Autodesk Fusion 360 part; units mm, degrees
sketch "Sketch1" plane through (0, 0, 0) normal (0, 0, 1) x (1, 0, 0)
  line L0 (7.5, 9) -> (-7.5, 9)
  line L1 (-7.5, 9) -> (-7.5, -9)
  line L2 (-7.5, -9) -> (2.5, -9)
  line L3 (7.5, -3) -> (7.5, 7)
  line L4 (2.5, -9) -> (7.5, -3)
  line L5 (5.5, 7) -> (7.5, 9)
  line L6 (7.5, 7) -> (7.5, 9)
  line L7 (5.5, 7) -> (-7.5, 7)
  dimension "d2" = 18
  dimension "d3" = 10
  dimension "d4" = 2
  dimension "d5" = 2
extrude "Extrude1" add sketch "Sketch1" along normal blind 6 contours L1 L2 L3 L4 L5 L6 L7
sketch "Sketch2" plane through (0, 0, 6) normal (0, 0, 1) x (-1, 0, 0)
  line L0 (-5.5, -7) -> (7.5, -7)
  line L1 (7.5, -7) -> (7.5, 9)
  line L2 (7.5, 9) -> (-2.5, 9)
  line L3 (-2.5, 9) -> (-7.5, 3)
  line L4 (-7.5, 3) -> (-7.5, -9)
  line L5 (-7.5, -9) -> (-5.5, -7)
  line L6 (-7.5, -9) -> (7.5, -9)
  line L7 (7.5, -9) -> (7.5, -7)
  dimension "d8" = 15
extrude "Extrude2" add sketch "Sketch2" along normal blind 6 and the other way blind 6 contours L0 L5 L6 L7
extrude "Extrude3" add 1 faces at (-2.5, 9, 6) along direction (0, 1, 0) blind 2
sketch "Sketch3" plane through (0, 7, 0) normal (0, -1, 0) x (1, 0, 0)
  line L0 (-7.5, 6) -> (5.5, 6)
  line L1 (5.5, 6) -> (5.5, 12)
  line L2 (5.5, 12) -> (-7.5, 12)
  line L3 (-7.5, 12) -> (-7.5, 6)
  line L4 (5.5, 12) -> (5.5, 10) construction
  line L5 (5.5, 10) -> (-0.5, 10) construction
  line L6 (-0.5, 10) -> (-7.5, 10)
  line L7 (-0.5, 10) -> (-0.5, 6)
extrude "Extrude4" add sketch "Sketch3" along normal blind 16 contours L0 L3 L6 L7
sketch "Sketch4" plane through (0, 0, 10) normal (0, 0, 1) x (-1, 0, 0)
  line L0 (0.5, -7) -> (7.5, -7)
  line L1 (7.5, -7) -> (7.5, 9)
  line L2 (7.5, 9) -> (0.5, 9)
  line L3 (0.5, 9) -> (0.5, -7)
  line L4 (7.5, 9) -> (5.5, 9)
  line L5 (5.5, 9) -> (5.5, 5)
  line L6 (0.5, -7) -> (0.5, -1)
  line L7 (5.5, 5) -> (0.5, -1)
  dimension "d17" = 2
  dimension "d18" = 6
extrude "Extrude5" cut sketch "Sketch4" against normal blind 4 contours L2 L3 L5 L7
sketch "Sketch5" plane through (0, 0, 10) normal (0, 0, 1) x (-1, 0, 0)
  line L0 (5.5, 9) -> (5.5, 5)
  line L1 (5.5, 5) -> (0.5, -1)
  line L2 (0.5, -1) -> (0.5, -7)
  line L3 (0.5, -7) -> (7.5, -7)
  line L4 (7.5, -7) -> (7.5, 9)
  line L5 (7.5, 9) -> (5.5, 9)
  line L6 (0.5, -1) -> (7.5, -1) construction
  circle A0 centre (4, -4) radius 1
  dimension "d21" = 2
extrude "Extrude6" cut sketch "Sketch5" against normal blind 6 contours A0
sketch "Sketch6" plane through (0, 7, 0) normal (0, -1, 0) x (1, 0, 0)
  line L0 (-0.5, 10) -> (-0.5, 6)
  line L1 (-0.5, 6) -> (5.5, 6)
  line L2 (5.5, 6) -> (5.5, 12)
  line L3 (5.5, 12) -> (-7.5, 12)
  line L4 (-7.5, 12) -> (-7.5, 10)
  line L5 (-7.5, 10) -> (-0.5, 10)
  line L6 (-0.5, 12) -> (-0.5, 11.8671) construction
  line L7 (-0.5, 11.8671) -> (-0.5, 10) construction
  circle A0 centre (2.5, 9) radius 1
  dimension "d24" = 2
extrude "Extrude7" cut sketch "Sketch6" against normal blind 3.5 contours A0
extrude "Extrude8" cut 1 faces at (2.6218, 10.5, 8.6897) along direction (0, 1, 0) blind 6
extrude "Extrude9" cut 1 faces at (-4.4091, 4.2521, 4) along direction (0, 0, -1) blind 58
Geometry: final body of the model. Coordinates: model frame, mm. A direction names the side the tool comes from. Round coordinates to 2 decimals unless told otherwise and drop trailing zeros. Loops run counter-clockwise (first coordinate to the right, second up) from the corner with the lowest first, then second, coordinate; pieces in that order, holes last. Notation, with made-up numbers: (37.5, -26.5) -> (90.5, -26.5) arc R30 ccw to (90.5, -3.5) -> close; hole circle Ø2 at (38.5, 39). An arc over 180 degrees is marked (long way). Use one line per item in the form item = value. Start each with the question number.
1) Section C-C on y = 4. Output: boundary loops of the cut face in (x, z).
2) Line query: L1, parallel to Y at x = -4, z = 5.5; L2, parallel to Z at x = 2.5, y = 9.25; L3, parallel to Y at x = 5, z = 10.75. Output: solid intervals per line, ascending.
3) Section D-D on z = 7.5. Output: boundary loops of the cut face in (x, y), then the cut area to 3 significant figures.
4) Draft query along X for faces 1 (the cylindrical face through (-3, 4, 5)), 2 (the flat face through (-5, 1, 10)), 3 (the flat face through (-3, -2, 8)). Return one class per face: released by +X, released by -X, zero draft, split by the parting line, or undercut.
5) Access query for faces 4 (the flat face through (-7.5, 1, 5)), 5 (the flat face through (6.5, 8, 9)). Directions: +Z, -Z, +X, -X, +Y, -Y. A direction counts if a zero-diameter tool reaches every point of the face in a straight line with its end or side. Return the directions, or none.
6) First-contact query: P1, Ø3, axis at x = 1.5, z = 9, coming from the -Y side; P2, Ø3, axis at y = 6.5, z = 9, coming from the +X side; P3, Ø5, axis at y = -7, z = 6, coming from the +X side. Flat tips, straight axial feed; report the tip coordinate or a pass-through.
7) Section B-B on x = -4. Output: boundary loops of the cut face in (y, z).
8) Section A-A on z = 9. Output: boundary loops of the cut face in (x, y), then the cut area to 3 significant figures.
Response:
q1.outline = (-7.5, 0) -> (-5, 0) -> (-5, 10) -> (-7.5, 10) -> close; (-3, 0) -> (7.5, 0) -> (7.5, 6) -> (-0.5, 6) -> (-0.5, 10) -> (-3, 10) -> close
q2.L1 = -9 to 3, 5 to 11
q2.L2 = 0 to 8, 10 to 12
q2.L3 = 7 to 11
q3.outline = (-7.5, -9) -> (-5.5, -9) -> (-5.5, -5) -> (-0.5, 1) -> (-0.5, 7) -> (5.5, 7) -> (7.5, 9) -> (7.5, 11) -> (-7.5, 11) -> close; hole circle Ø2 at (-4, 4)
q3.area = 132 mm^2
q4.face_1 = undercut
q4.face_2 = zero draft
q4.face_3 = released by +X
q5.face_4 = +Z, -Z, -X, +Y, -Y
q5.face_5 = +Z, +X, -Y
q6.P1 = 7
q6.P2 = 6.5
q6.P3 = 6.25
q7.outline = (-9, 0) -> (3, 0) -> (3, 10) -> (-3.2, 10) -> (-3.2, 6) -> (-9, 6) -> close; (5, 0) -> (11, 0) -> (11, 12) -> (7, 12) -> (7, 10) -> (5, 10) -> close
q8.outline = (-7.5, -9) -> (-5.5, -9) -> (-5.5, -5) -> (-0.5, 1) -> (-0.5, 7) -> (1.5, 7) -> (1.5, 11) -> (-7.5, 11) -> close; (3.5, 7) -> (5.5, 7) -> (7.5, 9) -> (7.5, 11) -> (3.5, 11) -> close; hole circle Ø2 at (-4, 4)
q8.area = 124 mm^2
